Check sheet for the drawn part. Datum: minimum x, y, z corner. Units: mm. A direction names the side the tool comes from. Coordinates: 2 decimals unless noted, no trailing zeros. Loops run counter-clockwise (first coordinate to the right, second up) from the corner with the lowest first, then second, coordinate; pieces in that order, holes last.
Q1. Sectioned sample at B-B (y = 14). Enter the section's corners in (x, z).
Q2. Mould release check, pull along Y, two halves, no side actions. Record for the marked faces 3, 4 and 5: +Y half, -Y half, draft (parallel to the pull), parting line (faces both ways), or undercut.
Q3. Access from +Z, -Z, +X, -X, +Y, -Y to the whole of each face (thin tool, end or side, straight path). Record for the marked faces 1 and 2.
Q4. Sectioned sample at D-D (x = 16). Enter the section's corners in (y, z), then the cut area to 3 significant figures.
Q5. Sectioned sample at A-A (z = 11.85). Enter the section's corners in (x, y).
Q6. Material ranges on probe 1 along X at (y, z) = (0.35, 30); probe 2 along X at (y, z) = (10, 34.5); probe 3 along Y at (x, z) = (12.25, 7), recorded low to high.
Q7. Go/stop test with flat-tipped pins: P1, Ø3, axis at x = 4, z = 45, coming from the -Y side; P2, Ø8, axis at y = 10.5, z = 8, coming from the -X side; P3, Ø4.5, axis at y = 7, z = 40, coming from the -X side; P4, Ø2.5, axis at x = 18, y = 2.5, coming from the +Z side. Record where each tip stops, or that it passes through.
Q8. Sectioned sample at C-C (z = 45). Enter the section's corners in (x, y).
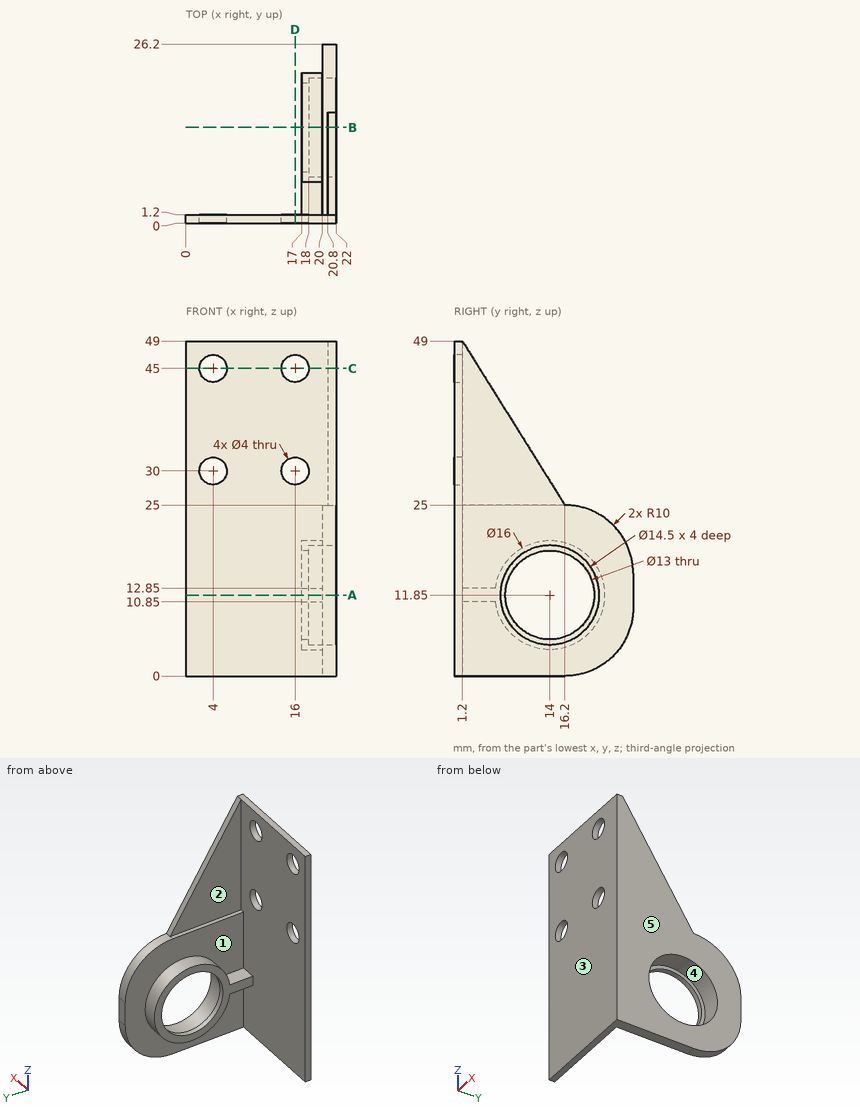
Geometry check:
1. outline: (17, 3.85) - (20, 3.85) - (20, 0) - (22, 0) - (22, 4.6) - (18, 4.6) - (18, 5.35) - (17, 5.35) - close; (17, 18.35) - (18, 18.35) - (18, 19.1) - (22, 19.1) - (22, 28.52) - (20.8, 28.52) - (20.8, 25) - (20, 25) - (20, 19.85) - (17, 19.85) - close
2. face 3: -Y half
2. face 4: undercut
2. face 5: draft
3. face 1: -X
3. face 2: +Z, -X, +Y
4. outline: (0, 0) - (1.2, 0) - (1.2, 28) - (0, 28) - close; (0, 32) - (1.2, 32) - (1.2, 43) - (0, 43) - close; (0, 47) - (1.2, 47) - (1.2, 49) - (0, 49) - close
4. area: 49.2 mm2
5. outline: (0, 0) - (22, 0) - (22, 6.75) - (18, 6.75) - (18, 7.5) - (17, 7.5) - (17, 1.2) - (0, 1.2) - close; (17, 20.5) - (18, 20.5) - (18, 21.25) - (22, 21.25) - (22, 26.2) - (20, 26.2) - (20, 22) - (17, 22) - close
6. probe 1: x = 0 to 2, 6 to 14, 18 to 22
6. probe 2: x = 20.8 to 22
6. probe 3: y = 0 to 1.2
7. P1: passes through
7. P2: stops at x = 17
7. P3: stops at x = 20.8
7. P4: stops at z = 12.85
8. outline: (0, 0) - (2, 0) - (2, 1.2) - (0, 1.2) - close; (6, 0) - (14, 0) - (14, 1.2) - (6, 1.2) - close; (18, 0) - (22, 0) - (22, 3.7) - (20.8, 3.7) - (20.8, 1.2) - (18, 1.2) - close
